Part model, mm, in its own coordinate system. A direction names the side the tool comes from. Give positions to 0.01 mm unless a question says otherwise; leave off trailing zeros. Write each loop counter-clockwise with the first axis right and the second up, starting at its lowest first coordinate (ties: lowest second). Pieces come first, ordered by that corner, then holes. Notation, with made-up numbers: M 56.25,72 L 89.25,72 A17 ccw 89.25,101 Z; hole C 4,87.5 d5. An arc over 180 degrees is marked long. Use CSV: the item, a comma, the result in double quotes. Start each with the question number.
1. Mould opens along X. For faces 6 (the face through (72, -21, -1)), 7 (the face through (1, -21, 72)), 8 (the face through (-67.9, 0, -69.5)), 9 (the face through (63.93, 0.76, 64)) say: pulls with the +X half, pulls with the -X half, needs draft (parallel to the pull), parting line crosses it, or undercut.
2. Band-saw the part on A-A, the plane y = -5. List the corners of the cut face in (x, z).
3. Drill centre lines: line 1 along X through (y, z) = (-5.75, 67.5); line 2 along X through (y, z) = (-27, -29.5). Where is each one in solid material? Low to high. Write a range as from..to.
4. Band-saw the part on C-C, the plane y = -26.5. List the corners of the cut face in (x, z), then the cut area to 3 significant figures.
5. Band-saw the part on D-D, the plane z = -51. List the corners of the cut face in (x, y).
6. Band-saw the part on B-B, the plane x = -22.5. List the corners of the cut face in (y, z), then the cut area to 3 significant figures.
7. Drop flat-ended pins along their axis: pin 1 Ø1.2 at (y, z) = (1, 69.5) entering from -X; pin 2 Ø3.5 at (x, y) = (70, -31) entering from +Z; pin 3 Ø1 at (x, z) = (-68, 67.5) entering from +Y. Give the stop position or say it passes through.
8. 3-axis set-ups, long thin cutter, end or side, ignore diameter. For faces 1 (the face through (1, -22, -75)), 2 (the face through (70, -21, -60)), 3 (the face through (67.6, 0, -69.5)), 4 (the face through (69, 0, 69)), 5 (the face through (-63.93, 0.76, -64)): which of +Z, -Z, +X, -X, +Y, -Y reach the whole face in a straight line?
from build123d import *

# Parameters (mm, degrees)
BOSS_EXTRUDE1_DEPTH = 46
BOSS_EXTRUDE2_START = 1.5
BOSS_EXTRUDE2_DEPTH = 1.5
SKETCH1_4_R         = 1.75
CUT_EXTRUDE1_DEPTH  = 13
BOSS_EXTRUDE3_START = -1.5
BOSS_EXTRUDE3_DEPTH = 1.5
FILLET1_R           = 2


with BuildPart() as part:
    # Sketch1 → Boss-Extrude1 (new body)
    with BuildSketch(Plane(origin=(0, 0, 0), x_dir=(1, 0, 0), z_dir=(0, 1, 0))):
        with BuildLine():
            Line((-67, -75), (67, -75))
            ThreePointArc((67, -75), (72.656854249, -72.656854249), (75, -67))
            Line((75, -67), (75, 67))
            ThreePointArc((75, 67), (72.656854249, 72.656854249), (67, 75))
            Line((67, 75), (-67, 75))
            ThreePointArc((-67, 75), (-72.656854249, 72.656854249), (-75, 67))
            Line((-75, 67), (-75, -67))
            ThreePointArc((-75, -67), (-72.656854249, -72.656854249), (-67, -75))
        make_face()
        with BuildLine():
            Line((-72, -60), (-72, 60))
            Line((-72, 60), (-67.5, 60))
            ThreePointArc((-67.5, 60), (-62.196699141, 62.196699141), (-60, 67.5))
            Line((-60, 67.5), (-60, 72))
            Line((-60, 72), (60, 72))
            Line((60, 72), (60, 67.5))
            ThreePointArc((60, 67.5), (62.196699141, 62.196699141), (67.5, 60))
            Line((67.5, 60), (72, 60))
            Line((72, 60), (72, -60))
            Line((72, -60), (67.5, -60))
            ThreePointArc((67.5, -60), (62.196699141, -62.196699141), (60, -67.5))
            Line((60, -67.5), (60, -72))
            Line((60, -72), (-60, -72))
            Line((-60, -72), (-60, -67.5))
            ThreePointArc((-60, -67.5), (-62.196699141, -62.196699141), (-67.5, -60))
            Line((-67.5, -60), (-72, -60))
        make_face(mode=Mode.SUBTRACT)
    extrude(amount=-BOSS_EXTRUDE1_DEPTH)

    # Sketch1_3 → Boss-Extrude2 (add)
    with BuildSketch(Plane(origin=(0, 0, 0), x_dir=(1, 0, 0), z_dir=(0, 1, 0)).offset(BOSS_EXTRUDE2_START)):
        with BuildLine():
            Line((-62.5, -67.5), (-62.5, -75))
            Line((-62.5, -75), (62.5, -75))
            Line((62.5, -75), (62.5, -67.5))
            ThreePointArc((62.5, -67.5), (63.964466094, -63.964466094), (67.5, -62.5))
            Line((67.5, -62.5), (75, -62.5))
            Line((75, -62.5), (75, 62.5))
            Line((75, 62.5), (67.5, 62.5))
            ThreePointArc((67.5, 62.5), (63.964466094, 63.964466094), (62.5, 67.5))
            Line((62.5, 67.5), (62.5, 75))
            Line((62.5, 75), (-62.5, 75))
            Line((-62.5, 75), (-62.5, 67.5))
            ThreePointArc((-62.5, 67.5), (-63.964466094, 63.964466094), (-67.5, 62.5))
            Line((-67.5, 62.5), (-75, 62.5))
            Line((-75, 62.5), (-75, -62.5))
            Line((-75, -62.5), (-67.5, -62.5))
            ThreePointArc((-67.5, -62.5), (-63.964466094, -63.964466094), (-62.5, -67.5))
        make_face()
        with BuildLine():
            Line((-67.5, -60), (-72, -60))
            Line((-72, -60), (-72, 60))
            Line((-72, 60), (-67.5, 60))
            ThreePointArc((-67.5, 60), (-62.196699141, 62.196699141), (-60, 67.5))
            Line((-60, 67.5), (-60, 72))
            Line((-60, 72), (60, 72))
            Line((60, 72), (60, 67.5))
            ThreePointArc((60, 67.5), (62.196699141, 62.196699141), (67.5, 60))
            Line((67.5, 60), (72, 60))
            Line((72, 60), (72, -60))
            Line((72, -60), (67.5, -60))
            ThreePointArc((67.5, -60), (62.196699141, -62.196699141), (60, -67.5))
            Line((60, -67.5), (60, -72))
            Line((60, -72), (-60, -72))
            Line((-60, -72), (-60, -67.5))
            ThreePointArc((-60, -67.5), (-62.196699141, -62.196699141), (-67.5, -60))
        make_face(mode=Mode.SUBTRACT)
    extrude(amount=-BOSS_EXTRUDE2_DEPTH)

    # Sketch1_4 → Cut-Extrude1 (cut)
    with BuildSketch(Plane(origin=(0, 0, 0), x_dir=(1, 0, 0), z_dir=(0, 1, 0))):
        with Locations(Location((-67.5, 67.5, 0), (0, 0, 270))):
            Circle(SKETCH1_4_R)
        with Locations(Location((-67.5, -67.5, 0), (0, 0, 270))):
            Circle(SKETCH1_4_R)
        with Locations(Location((67.5, -67.5, 0), (0, 0, 270))):
            Circle(SKETCH1_4_R)
        with Locations(Location((67.5, 67.5, 0), (0, 0, 270))):
            Circle(SKETCH1_4_R)
    extrude(amount=-CUT_EXTRUDE1_DEPTH, mode=Mode.SUBTRACT)

    # Sketch2 → Boss-Extrude3 (add)
    with BuildSketch(Plane.XZ.offset(46).offset(BOSS_EXTRUDE3_START)):
        with BuildLine():
            Line((-75, 67), (-75, -67))
            ThreePointArc((-75, -67), (-72.656854249, -72.656854249), (-67, -75))
            Line((-67, -75), (67, -75))
            ThreePointArc((67, -75), (72.656854249, -72.656854249), (75, -67))
            Line((75, -67), (75, 67))
            ThreePointArc((75, 67), (72.656854249, 72.656854249), (67, 75))
            Line((67, 75), (-67, 75))
            ThreePointArc((-67, 75), (-72.656854249, 72.656854249), (-75, 67))
        make_face()
    extrude(amount=BOSS_EXTRUDE3_DEPTH)

    # Fillet1
    fillet1_edges = [part.edges().sort_by_distance(p)[0] for p in [
        (-75, 0.75, -62.5),
        (-75, 0.75, 62.5),
        (-62.5, 0.75, 75),
        (62.5, 0.75, 75),
        (75, 0.75, 62.5),
        (75, 0.75, -62.5),
        (62.5, 0.75, -75),
        (-62.5, 0.75, -75),
    ]]
    fillet(fillet1_edges, radius=FILLET1_R)


solid = part.part
Output:
1,face 6,"undercut"
1,face 7,"undercut"
1,face 8,"needs draft"
1,face 9,"pulls with the +X half"
2,outline,"M -75,-67 A8 ccw -67,-75 L 67,-75 A8 ccw 75,-67 L 75,67 A8 ccw 67,75 L -67,75 A8 ccw -75,67 Z; hole M -72,-60 L -67.5,-60 A7.5 cw -60,-67.5 L -60,-72 L 60,-72 L 60,-67.5 A7.5 cw 67.5,-60 L 72,-60 L 72,60 L 67.5,60 A7.5 cw 60,67.5 L 60,72 L -60,72 L -60,67.5 A7.5 cw -67.5,60 L -72,60 Z; hole C -67.5,-67.5 d3.5; hole C -67.5,67.5 d3.5; hole C 67.5,-67.5 d3.5; hole C 67.5,67.5 d3.5"
3,line 1,"x = -74.98..-69.25, -65.75..-60, 60..65.75, 69.25..74.98"
3,line 2,"x = -75..-72, 72..75"
4,outline,"M -75,-67 A8 ccw -67,-75 L 67,-75 A8 ccw 75,-67 L 75,67 A8 ccw 67,75 L -67,75 A8 ccw -75,67 Z; hole M -72,-60 L -67.5,-60 A7.5 cw -60,-67.5 L -60,-72 L 60,-72 L 60,-67.5 A7.5 cw 67.5,-60 L 72,-60 L 72,60 L 67.5,60 A7.5 cw 60,67.5 L 60,72 L -60,72 L -60,67.5 A7.5 cw -67.5,60 L -72,60 Z"
4,area,"2,240 mm²"
5,outline,"M -75,-46 L 75,-46 L 75,1.5 L 72,1.5 L 72,-44.5 L -72,-44.5 L -72,1.5 L -75,1.5 Z"
6,outline,"M -46,-75 L 1.5,-75 L 1.5,-72 L -44.5,-72 L -44.5,72 L 1.5,72 L 1.5,75 L -46,75 Z"
6,area,"501 mm²"
7,pin 1,"stops at x = -62.5"
7,pin 2,"stops at z = 74.9"
7,pin 3,"stops at y = -13"
8,face 1,"-Z, +X, -X, +Y, -Y"
8,face 2,"+Y"
8,face 3,"-Z, +X, +Y"
8,face 4,"+Z, +X, +Y"
8,face 5,"-Z, -X, +Y"
